Geometry: final body of the model. Coordinates: model frame, mm. A direction names the side the tool comes from. Coordinates: 2 decimals unless noted, no trailing zeros. Loops run counter-clockwise (first coordinate to the right, second up) from the corner with the lowest first, then second, coordinate; pieces in that order, holes last. Notation, with made-up numbers: (29.5, -18) -> (43.5, -18) arc R27 cw to (43.5, 4) -> close; hole circle Ø3 at (31, -25). An arc over 180 degrees is marked (long way). One line per item, written item: value. Start each with the question number.
from build123d import *

# Parameters (mm, degrees)
F0_R      = 15.875
F1_DEPTH  = 31.75
F2_R      = 11.049
F3_DEPTH  = 12.7
F5_D      = 10.71626
F5_DEPTH  = 18.5615384615
F5_TIP    = 3.2194893086
F7_D      = 3.175
F7_DEPTH  = 6.35
F7_TIP    = 0.9538662327
F8_R      = 0.127
F10_D     = 14.68374
F10_DEPTH = 25.4
F10_TIP   = 4.411440553


with BuildPart() as f1:
    # F0 (on Top) → F1 (new body)
    with BuildSketch(Plane.XY):
        Circle(F0_R)
    extrude(amount=F1_DEPTH)

    # F2 (on face) → F3 (join)
    with BuildSketch(Plane.XY.offset(31.75)):
        Circle(F2_R)
    extrude(amount=F3_DEPTH)

    # F5
    with Locations(Plane.XY.offset(44.45)):
        with Locations((0, 0)):
            Hole(F5_D / 2, depth=F5_DEPTH)
            with Locations((0, 0, -(F5_DEPTH + F5_TIP / 2))):  # 118° drill point
                Cone(0, F5_D / 2, F5_TIP, mode=Mode.SUBTRACT)

    # F7
    with Locations(Plane.XY.offset(31.75)):
        with Locations((-12.7611987248, 0), (12.7453794703, 0)):
            Hole(F7_D / 2, depth=F7_DEPTH)
            with Locations((0, 0, -(F7_DEPTH + F7_TIP / 2))):  # 118° drill point
                Cone(0, F7_D / 2, F7_TIP, mode=Mode.SUBTRACT)

    # F8
    f8_edges = [f1.edges().sort_by_distance(p)[0] for p in [
        (-11.049, 0, 44.45),
        (-15.875, 0, 31.75),
    ]]
    fillet(f8_edges, radius=F8_R)

    # F10
    with Locations(Plane(origin=(0, 0, 0), x_dir=(1, 0, 0), z_dir=(0, 0, -1))):
        with Locations((0, 0)):
            Hole(F10_D / 2, depth=F10_DEPTH)
            with Locations((0, 0, -(F10_DEPTH + F10_TIP / 2))):  # 118° drill point
                Cone(0, F10_D / 2, F10_TIP, mode=Mode.SUBTRACT)


solid = f1.part
1. Set-up query: faces 4 (the face through (-2.472, -4.754, 35.396)), 5 (the face through (14.33, 0.07, 28.53)). Return all of +Z, -Z, +X, -X, +Y, -Y with unobstructed straight access to the full face (end or side cutting, diameter ignored); none if empty.
2. Draft query along X for faces 1 (the face through (1.592, 7.167, 12.878)), 2 (the face through (5, 3, 44.45)), 3 (the face through (-3.441, -15.497, 15.59)). Return one class per face: released by +X, released by -X, zero draft, split by the parting line, or undercut.
3. Section B-B on z = 32.5. Return the cut outline in (x, y), plus the area to 3 significant figures.
4. Pin query (flat end, axial travel): pin 1 Ø5 at (x, y) = (-12.76, 0) entering from +Z; pin 2 Ø3 at (x, z) = (9, 15.5) entering from +Y; pin 3 Ø10 at (x, z) = (9, 12.5) entering from +Y; pin 4 Ø1 at (x, z) = (1.5, 11) entering from -Y. Return the tip coordinate at first contact, or that it passes through.
5. Section A-A on x = 0. Return the cut outline in (y, z) (3 decimals).
6. Line query: L1, parallel to Y at x = 0, z = 32.25; L2, parallel to Y at x = 3, z = 11; L3, parallel to X at y = -4.5, z = 28. Output: solid intervals per line, ascending. Write a range as [from, to].
7. Section C-C on z = 7.5. Return the cut outline in (x, y) (3 decimals), plus the area to 3 significant figures.
Checks:
1. face 4: +Z, -Z
1. face 5: +Z
2. face 1: undercut
2. face 2: zero draft
2. face 3: split by the parting line
3. outline: circle Ø22.1 at (0, 0); hole circle Ø10.72 at (0, 0)
3. area: 293 mm²
4. pin 1: z = 44.45
4. pin 2: y = 13.99
4. pin 3: y = 15.36
4. pin 4: y = -15.84
5. outline: (-15.875, 0) -> (-7.342, 0) -> (-7.342, 25.4) -> (-5.358, 26.592) -> (-5.358, 44.45) -> (-10.922, 44.45) arc R0.127 ccw to (-11.049, 44.323) -> (-11.049, 31.75) -> (-15.748, 31.75) arc R0.127 ccw to (-15.875, 31.623) -> close; (5.358, 26.592) -> (7.342, 25.4) -> (7.342, 0) -> (15.875, 0) -> (15.875, 31.623) arc R0.127 ccw to (15.748, 31.75) -> (11.049, 31.75) -> (11.049, 44.323) arc R0.127 ccw to (10.922, 44.45) -> (5.358, 44.45) -> close
6. L1: [-11.05, -5.36], [5.36, 11.05]
6. L2: [-15.59, -6.7], [6.7, 15.59]
6. L3: [-15.22, -2.91], [2.91, 15.22]
7. outline: circle Ø31.75 at (0, 0); hole circle Ø14.684 at (0, 0)
7. area: 622 mm²
